Read the model definition and answer for the solid it produces. Units are mm, in the model's axes. A direction names the side the tool comes from. Coordinates: 2 decimals unless noted, no trailing zeros. Write each loop counter-clockwise with the first axis right and the second up, starting at its lowest first coordinate (ties: lowest second). Pieces come first, ordered by that corner, then holes.
Item 1: Section A-A (x = -15) is taken. Give the vertices of the cut face in (y, z).
Item 2: Determine the mould class of faces 1 (the face through (-1.995, 6.691, 4.028)), 2 (the face through (3, 9.95, 7)), 3 (the face through (4.38, -9.37, 4.06)) for opening direction X: released by +X, released by -X, zero draft, split by the parting line, or undercut.
Item 3: Section B-B (y = -9) is taken. Give the vertices of the cut face in (x, z).
Item 4: Section C-C (z = 4.25) is taken. State how many separate pieces and enclosed holes the cut face has, then the cut area to 3 significant figures.
Item 5: A tool of negligible diameter and unlimited length cuts with its end or side. For faces 4 (the face through (-29.66, -16.58, 3.94)), 5 (the face through (3, -9.95, 7)), 6 (the face through (-2.04, -6.59, 4.03)), 7 (the face through (-26.74, 13.96, 4.06)), from which of +Z, -Z, +X, -X, +Y, -Y can it reach the whole face along a straight path? Write none if from no direction.
Item 6: Each of these flat-tipped pins is pushed along its axis until it touches: P1, Ø0.5, axis at x = 3, z = 2, coming from the +Y side; P2, Ø4, axis at x = -3, z = 3.5, coming from the -Y side; P3, Ø1, axis at x = -12.5, y = -13, coming from the +Z side; P4, Ø2, axis at x = -9, z = 5.5, coming from the +Y side. Where does it stop, or does it pass through?
Item 7: Straight lines are drawn through the part: probe 1 along Z at (x, y) = (-2, 3); probe 2 along Y at (x, z) = (-17.5, 5.5); probe 3 along Y at (x, z) = (-12.5, 4.25). For each, find the intervals that lie inside material, in ascending order.
Item 8: Section D-D (z = 1) is taken. Give the vertices of the cut face in (x, y) (3 decimals), then the cut area to 3 significant figures.
from build123d import *

# Parameters (mm, degrees)
F1_DEPTH = 8
F2_R     = 5
F3_R     = 1
F4_R     = 10
F7_DEPTH = 4
F8_R     = 1


# Not quite as in the source:
# - a feature names something its author has since deleted; it is built from what else it names


with BuildPart() as f1:
    # F0 (on Top) → F1 (new body)
    with BuildSketch(Plane.XY):
        with BuildLine():
            ThreePointArc((-2.9227996939, -0.1596333839), (-11.2678550126, -13.4433261015), (-26.890906557, -12.0232201439))
            Line((-26.890906557, -12.0232201439), (-31.1837848276, -19.0931353718))
            Line((-31.1837848276, -19.0931353718), (-22.9890488593, -17.2720731705))
            ThreePointArc((-22.9890488593, -17.2720731705), (-11.7519193442, -16.909486057), (-2.9219502426, -9.9498743711))
            Line((-2.9219502426, -9.9498743711), (6.0116767822, -9.9498743711))
            ThreePointArc((6.0116767822, -9.9498743711), (1.0780497574, 0), (6.0116767822, 9.9498743711))
            Line((6.0116767822, 9.9498743711), (-2.9219502426, 9.9498743711))
            ThreePointArc((-2.9219502426, 9.9498743711), (-11.7519193442, 16.909486057), (-22.9890488593, 17.2720731705))
            Line((-22.9890488593, 17.2720731705), (-31.1837848276, 19.0931353718))
            Line((-31.1837848276, 19.0931353718), (-26.890906557, 12.0232201439))
            ThreePointArc((-26.890906557, 12.0232201439), (-11.3609432233, 13.4890024425), (-2.9264400932, 0.3669814152))
            Line((-2.9264400932, 0.3669814152), (-2.9219502426, 0.3647975664))
            Line((-2.9219502426, 0.3647975664), (-2.9219502426, -3.27e-08))
            Line((-2.9219502426, -3.27e-08), (-2.9219502426, -0.1592372783))
            Line((-2.9219502426, -0.1592372783), (-2.9227996939, -0.1596333839))
        make_face()
        with BuildLine():
            ThreePointArc((-2.9219502426, -3.27e-08), (-2.922162607, -0.0798178383), (-2.9227996939, -0.1596333839))
            Line((-2.9227996939, -0.1596333839), (-2.9219502426, -0.1592372783))
            Line((-2.9219502426, -0.1592372783), (-2.9219502426, -3.27e-08))
        make_face()
        with BuildLine():
            ThreePointArc((-2.9264400932, 0.3669814152), (-2.923072747, 0.1835044236), (-2.9219502426, -3.27e-08))
            Line((-2.9219502426, -3.27e-08), (-2.9219502426, 0.3647975664))
            Line((-2.9219502426, 0.3647975664), (-2.9264400932, 0.3669814152))
        make_face()
    extrude(amount=F1_DEPTH)

    # F2
    f2_edges = [f1.edges().sort_by_distance(p)[0] for p in [
        (-26.890907, 12.02322, 4),
        (-26.890907, -12.02322, 4),
    ]]
    fillet(f2_edges, radius=F2_R)

    # F3
    f3_edges = [f1.edges().sort_by_distance(p)[0] for p in [
        (-31.183785, -19.093135, 4),
        (-31.183785, 19.093135, 4),
    ]]
    fillet(f3_edges, radius=F3_R)

    # F4
    f4_edges = [f1.edges().sort_by_distance(p)[0] for p in [
        (-2.92195, 9.949874, 4),
        (-2.92195, -9.949874, 4),
        (-22.989049, 17.272073, 4),
        (-22.989049, -17.272073, 4),
    ]]
    fillet(f4_edges, radius=F4_R)

    # F6 (on offset) → F7 (cut)
    with BuildSketch(Plane.XY.offset(6)):
        with BuildLine():
            ThreePointArc((11.3967054025, -13.8123607251), (-0.7746921386, -2.0181552322), (7.4959259895, 12.7751904709))
            Line((7.4959259895, 12.7751904709), (2.6926121721, 12.7751904709))
            ThreePointArc((2.6926121721, 12.7751904709), (-3.3979094134, -0.8877509035), (4.1336827916, -13.8123607251))
            Line((4.1336827916, -13.8123607251), (11.3967054025, -13.8123607251))
        make_face()
    extrude(amount=-F7_DEPTH, mode=Mode.SUBTRACT)

    # F8
    f8_edges = [f1.edges().sort_by_distance(p)[0] for p in [
        (6.011677, 9.949874, 4),
        (6.011677, -9.949874, 4),
    ]]
    fillet(f8_edges, radius=F8_R)


solid = f1.part
Established:
1. outline: (-17.76, 0) - (-14.71, 0) - (-14.71, 8) - (-17.76, 8) - close; (14.71, 0) - (17.76, 0) - (17.76, 8) - (14.71, 8) - close
2. face 1: undercut
2. face 2: zero draft
2. face 3: released by +X
3. outline: (-5.92, 0) - (4.47, 0) - (4.47, 8) - (-5.92, 8) - close; hole (-0.73, 2) - (2.38, 2) - (2.38, 6) - (-0.73, 6) - close
4. separate pieces: 3
4. enclosed holes: 0
4. area: 257 mm2
5. face 4: +Z, -Z, -X
5. face 5: +Z, -Z, +X, -Y
5. face 6: none
5. face 7: +Z, -Z
6. P1: stops at y = 9.95
6. P2: stops at y = -12.55
6. P3: passes through
6. P4: stops at y = 16.16
7. probe 1: z = 0 to 2, 6 to 8
7. probe 2: y = -18 to -14.99, 14.99 to 18
7. probe 3: y = -17.16 to -13.99, 13.99 to 17.16
8. outline: (-29.967, -17.089) arc R1 ccw to (-28.895, -18.585) - (-25.212, -17.766) arc R10 cw to (-21.214, -17.696) arc R18 ccw to (-5.292, -12.825) arc R10 cw to (1.725, -9.95) - (3.471, -9.95) arc R1 ccw to (4.22, -8.287) arc R12.5 cw to (4.22, 8.287) arc R1 ccw to (3.471, 9.95) - (1.725, 9.95) arc R10 cw to (-5.292, 12.825) arc R18 ccw to (-21.214, 17.696) arc R10 cw to (-25.212, 17.766) - (-28.895, 18.585) arc R1 ccw to (-29.967, 17.089) - (-29.354, 16.08) arc R5 ccw to (-23.291, 14.006) arc R15 cw to (-2.922, 0) arc R15 cw to (-2.923, -0.16) arc R15 cw to (-23.291, -14.006) arc R5 ccw to (-29.354, -16.08) - close
8. area: 309 mm2
